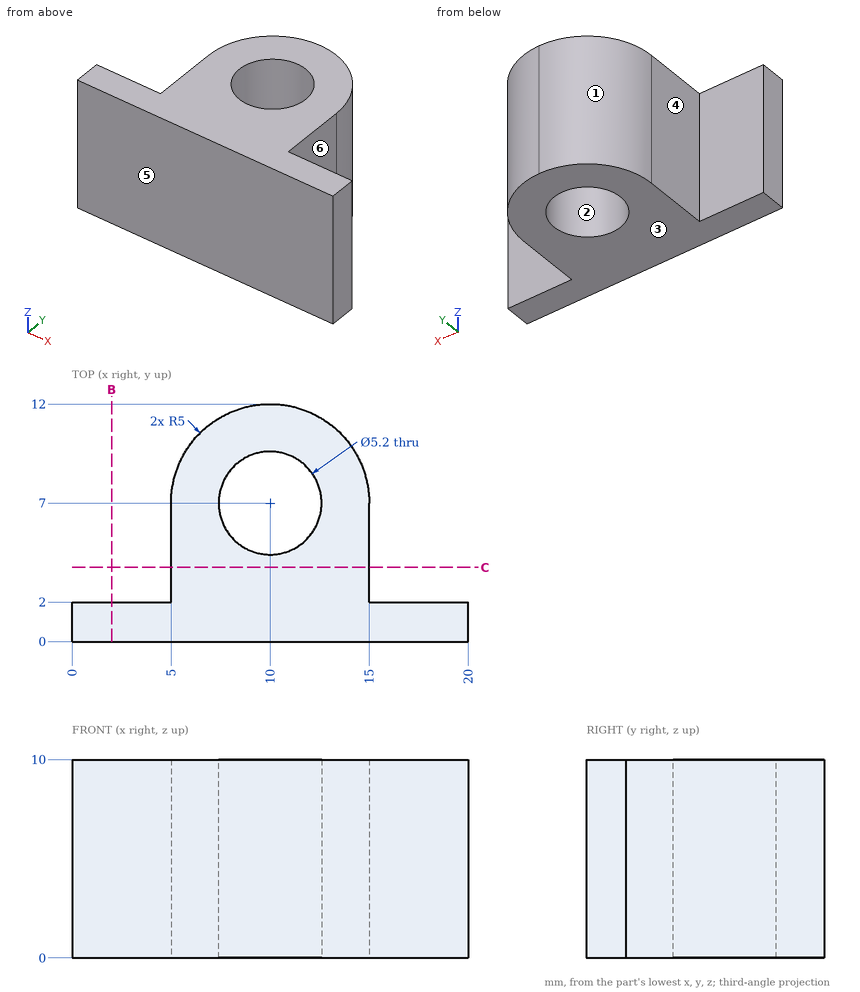
Drawing for the job (mm, zero at the part's lowest x, y, z). A direction names the side the tool comes from. Give positions to 0.01 mm unless a question says otherwise; leave off trailing zeros. Order: outer loops, then holes, each group sorted by start corner. A loop starts at its lowest first (then second) coordinate and runs counter-clockwise, first axis right, second up. Notation, with made-up numbers: (81.5, 69) -> (107.5, 69) arc R31 ccw to (107.5, 94) -> close; hole circle Ø5 at (31.5, 29.25). An arc over 180 degrees is marked (long way). Use one line per item in the form item = value.
(1) Drill centre lines: line 1 (Y direction, x = 10, z = 4); line 2 (Y direction, x = 8, z = 7.5); line 3 (X direction, y = 8, z = 0.75). Where is each one in solid material? Low to high. Write a range as from..to.
Solution:
line_1 = 0..4.4, 9.6..12
line_2 = 0..5.34, 8.66..11.58
line_3 = 5.1..7.6, 12.4..14.9
(2) Tool access for the marked faces 4, 5 and 6: list every direction of +Z, -Z, +X, -X, +Y, -Y with a clear straight run to the whole face (end or side of a thin tool).
Solution:
face_4 = +Z, -Z, -X, +Y
face_5 = +Z, -Z, +X, -X, -Y
face_6 = +Z, -Z, +X, +Y
(3) Saw through at B-B (x = 2). Write the cut outline in (y, z), then the cut area to 3 significant figures.
Solution:
outline = (0, 0) -> (2, 0) -> (2, 10) -> (0, 10) -> close
area = 20.0 mm²
(4) Saw through at C-C (y = 3.75). Write the cut outline in (x, z).
Solution:
outline = (5, 0) -> (15, 0) -> (15, 10) -> (5, 10) -> close
(5) Flat gauge pins, fed straight in: P1, Ø6, axis at x = 4.5, y = 8.5, coming from the -Z side; P2, Ø4, axis at y = 5, z = 6.5, coming from the -X side; P3, Ø5, axis at y = 10.5, z = 6.5, coming from the -X side; P4, Ø1.5, axis at x = 18, z = 4, coming from the +Y side. Where does each tip first touch, or does it go through?
Solution:
P1 = 0
P2 = 5
P3 = 5.1
P4 = 2
(6) Pull direction X, two halves, no side cores. Call the marked faces 1, 2 and 3: +X half, -X half, draft (parallel to the pull), parting line (faces both ways), or undercut.
Solution:
face_1 = -X half
face_2 = undercut
face_3 = draft
